Could you check a few things on this model? Use its own coordinates, in mm. Coordinates: 2 decimals unless noted, no trailing zeros. Write each loop counter-clockwise with the first axis right and the second up, starting at its lowest first coordinate (ties: lowest second). Pieces come first, ordered by that corner, then holes. Notation, with made-up numbers: (80, 82) - (86, 82) arc R9 cw to (86, 92) - close; hole circle Ø4 at (52, 69.5). An arc over 180 degrees is marked (long way). Write item = value, one per line. Start each with the question number.
```python
from build123d import *

# Parameters (mm, degrees)
EXTRUDE_1_DEPTH          = 10
SKETCH_2_R               = 16
CUT_EXTRUDE_1_DEPTH      = 10
SKETCH_3_R               = 5
CUT_EXTRUDE_2_DEPTH      = 10
SKETCH_6_R               = 2
CUT_EXTRUDE_4_DEPTH      = 10
PATTERN_CIRCULAR_1_COUNT = 4
FILLET_1_R               = 0.5


with BuildPart() as part:
    # 草图1 → 凸台-拉伸1 (new body)
    with BuildSketch(Plane.XY):
        Polygon((50, -85), (-50, -85), (-50, -20), (-50, 85), (50, 85), (50, 0), align=None)
    extrude(amount=EXTRUDE_1_DEPTH)

    # 草图2 → 切除-拉伸1 (cut)
    with BuildSketch(Plane.XY.offset(10)):
        Circle(SKETCH_2_R)
    extrude(amount=-CUT_EXTRUDE_1_DEPTH, mode=Mode.SUBTRACT)

    # 草图3 → 切除-拉伸2 (cut)
    with BuildSketch(Plane.XY.offset(10)):
        with Locations((0, -72)):
            Circle(SKETCH_3_R)
        with Locations((35, -72)):
            Circle(SKETCH_3_R)
        with Locations((-35, -72)):
            Circle(SKETCH_3_R)
    cut_extrude_2 = extrude(amount=-CUT_EXTRUDE_2_DEPTH, mode=Mode.SUBTRACT)

    # 草图6 → 切除-拉伸4 (cut)
    with BuildSketch(Plane.XY.offset(10)):
        with Locations((0, 21)):
            Circle(SKETCH_6_R)
    cut_extrude_4 = extrude(amount=-CUT_EXTRUDE_4_DEPTH, mode=Mode.SUBTRACT)

    # 阵列(圆周)1: 切除-拉伸4 ×4 about axis
    pattern_circular_1_axis = Axis((0, 0, 0), (0, 0, 1))
    for i in range(1, PATTERN_CIRCULAR_1_COUNT):
        add(cut_extrude_4.rotate(pattern_circular_1_axis, i * 360 / PATTERN_CIRCULAR_1_COUNT), mode=Mode.SUBTRACT)

    # 镜向1: 切除-拉伸2 across plane
    add(cut_extrude_2.mirror(Plane.ZX), mode=Mode.SUBTRACT)

    # 圆角1
    fillet_1_edges = [part.edges().sort_by_distance(p)[0] for p in [
        (50, -85, 5),
        (-50, -85, 5),
        (-50, 85, 5),
        (50, 85, 5),
        (-50, 0, 10),
        (0, -85, 10),
        (50, 0, 10),
        (50, 0, 0),
        (0, -85, 0),
        (-50, 0, 0),
        (0, 85, 0),
        (0, 85, 10),
    ]]
    fillet(fillet_1_edges, radius=FILLET_1_R)


solid = part.part
```
1) Suppose I cut it at C-C on z = 2. State how many separate pieces and enclosed holes the cut face has, plus the area to 3 significant figures.
2) Suppose I cut it at A-A on x = 21. Please give me the cut outline in (y, z), plus the area to 3 significant figures.
3) Suppose I cut it at D-D on x = 0. Please give me the cut outline in (y, z), plus the area to 3 significant figures.
4) For P1, Ø2.5, axis at x = 0, y = 21, coming from the -Z side, with a flat end and sliding along its axis, tell me the tip position at first contact or that it passes through.
5) If I drill on probe 1 along Y at (x, z) = (-35, 5); probe 2 along X at (y, z) = (72, 5); probe 3 along Y at (x, z) = (0, 7.5), over which ranges is the centre line in solid material (lowest first)? Write a range as [from, to].
6) Suppose I cut it at B-B on y = 21. Please give me the cut outline in (x, z).
7) Thinking about a two-plate mould opening in Y: for faces 1 (the flat face through (-1, 85, 5)), 2 (the cylindrical face through (-23, 0, 5)), 3 (the flat face through (1, -18, 0)), which applies, +Y half, -Y half, draft (parallel to the pull), parting line (faces both ways), or undercut?
Reply:
q1.separate_pieces = 1
q1.enclosed_holes = 11
q1.area = 15,700 mm^2
q2.outline = (-85, 0.5) arc R0.5 ccw to (-84.5, 0) - (-2, 0) - (-2, 10) - (-84.5, 10) arc R0.5 ccw to (-85, 9.5) - close; (2, 0) - (84.5, 0) arc R0.5 ccw to (85, 0.5) - (85, 9.5) arc R0.5 ccw to (84.5, 10) - (2, 10) - close
q2.area = 1,660 mm^2
q3.outline = (-85, 0.5) arc R0.5 ccw to (-84.5, 0) - (-77, 0) - (-77, 10) - (-84.5, 10) arc R0.5 ccw to (-85, 9.5) - close; (-67, 0) - (-23, 0) - (-23, 10) - (-67, 10) - close; (-19, 0) - (-16, 0) - (-16, 10) - (-19, 10) - close; (16, 0) - (19, 0) - (19, 10) - (16, 10) - close; (23, 0) - (67, 0) - (67, 10) - (23, 10) - close; (77, 0) - (84.5, 0) arc R0.5 ccw to (85, 0.5) - (85, 9.5) arc R0.5 ccw to (84.5, 10) - (77, 10) - close
q3.area = 1,100 mm^2
q4.P1 = through
q5.probe_1 = [-85, -77], [-67, 67], [77, 85]
q5.probe_2 = [-50, -40], [-30, -5], [5, 30], [40, 50]
q5.probe_3 = [-85, -77], [-67, -23], [-19, -16], [16, 19], [23, 67], [77, 85]
q6.outline = (-50, 0.5) arc R0.5 ccw to (-49.5, 0) - (-2, 0) - (-2, 10) - (-49.5, 10) arc R0.5 ccw to (-50, 9.5) - close; (2, 0) - (49.5, 0) arc R0.5 ccw to (50, 0.5) - (50, 9.5) arc R0.5 ccw to (49.5, 10) - (2, 10) - close
q7.face_1 = +Y half
q7.face_2 = undercut
q7.face_3 = draft
